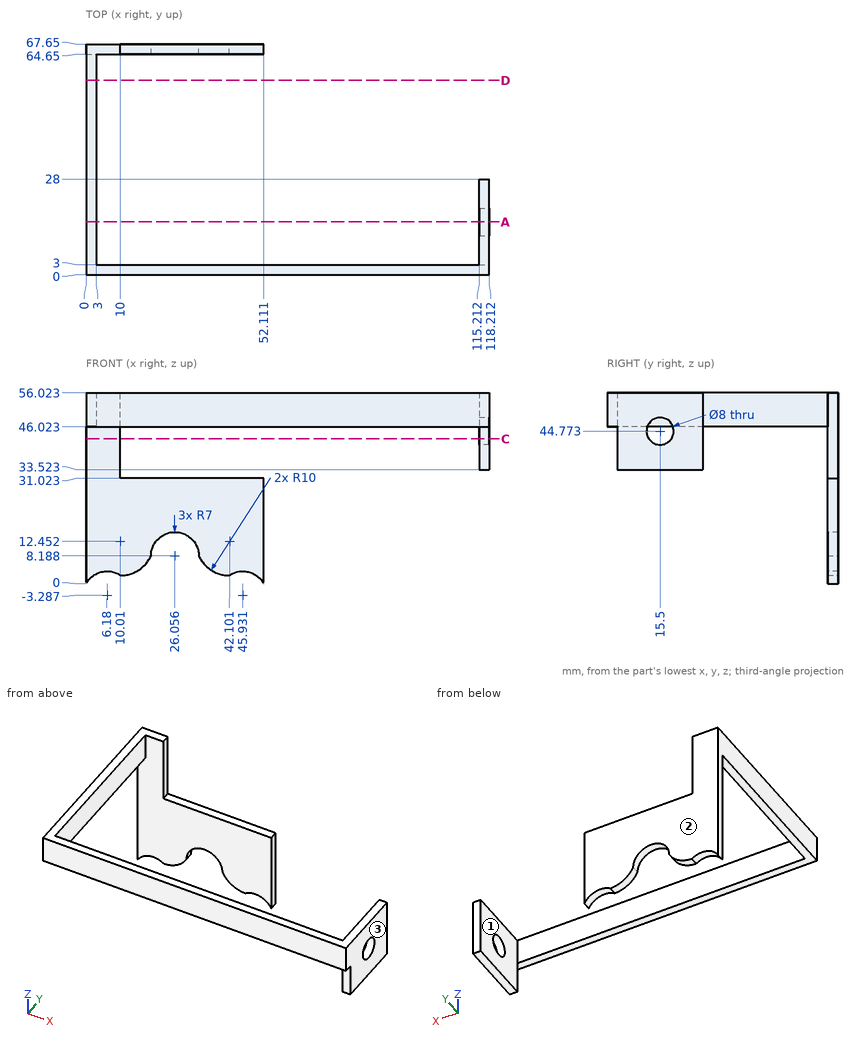
Check sheet for the drawn part. Datum: minimum x, y, z corner. Units: mm. Coordinates: 2 decimals unless noted, no trailing zeros. Order: outer loops, then holes, each group sorted by start corner. A loop starts at its lowest first (then second) coordinate and runs counter-clockwise, first axis right, second up. Notation, with made-up numbers: M 40,-30.75 L 80,-30.75 A13 ccw 80,-9.75 Z; hole C 83,24.25 d10. An arc over 180 degrees is marked long. One line per question, with ' | ' between items. Start each with the question number.
Item 1: Material ranges on L1, parallel to Y at x = 7.5, z = 50.5; L2, parallel to X at y = 21, z = 37; L3, parallel to X at y = 30.5, z = 51, recorded low to high. Write a range as [from, to].
Item 2: Cross-section at C-C on z = 42.5. Enter the section's corners in (x, y).
Item 3: Cross-section at D-D on y = 57. Enter the section's corners in (x, z).
Item 4: Draft check along X on the marked faces 1, 2 and 3. Enter one of: pulls with the +X half, pulls with the -X half, needs draft (parallel to the pull), parting line crosses it, or undercut.
Item 5: Cross-section at A-A on y = 15.5. Enter the section's corners in (x, z).
Item 6: Gauge pin test, flat ends, axial feed: pin 1 (1.5 mm diameter, centred on x = 22, y = 66, fed in from +Z); pin 2 (5 mm diameter, centred on y = 47.5, z = 53, fed in from +X); pin 3 (3.5 mm diameter, centred on x = 116.5, z = 40, fed in from +Y); pin 4 (10 mm diameter, centred on y = 27, z = 28, fed in from -X). Record the tip position at first contact, or that the pin passes through.
Findings:
1) L1: y = [0, 3], [64.65, 67.65] | L2: x = [115.21, 118.21] | L3: x = [0, 3]
2) outline: M 0,64.65 L 10,64.65 L 10,67.65 L 0,67.65 Z; M 115.21,3 L 118.21,3 L 118.21,12.21 L 115.21,12.21 Z; M 115.21,18.79 L 118.21,18.79 L 118.21,28 L 115.21,28 Z
3) outline: M 0,46.02 L 3,46.02 L 3,56.02 L 0,56.02 Z
4) face 1: undercut | face 2: needs draft | face 3: pulls with the +X half
5) outline: M 0,46.02 L 3,46.02 L 3,56.02 L 0,56.02 Z; M 115.21,33.52 L 118.21,33.52 L 118.21,40.77 L 115.21,40.77 Z; M 115.21,48.77 L 118.21,48.77 L 118.21,56.02 L 115.21,56.02 Z
6) pin 1: stops at z = 31.02 | pin 2: stops at x = 3 | pin 3: stops at y = 28 | pin 4: passes through
